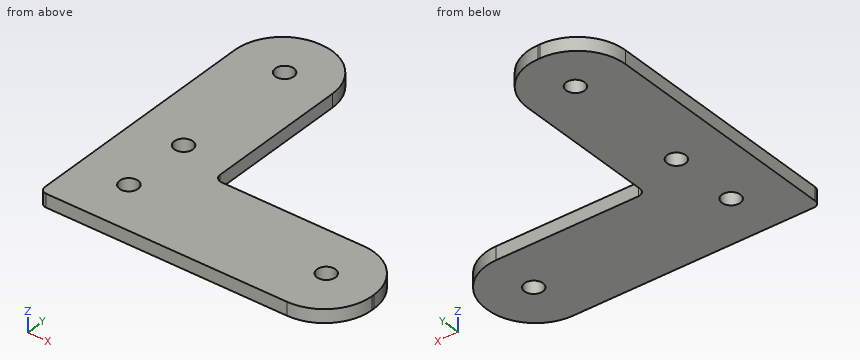
from build123d import *

# Parameters (mm, degrees)
BOSS_EXTRUDE1_DEPTH      = 3
FILLET4_R                = 21.5
FILLET5_R                = 3.4
FILLET6_R                = 3
F_5_16_CLEARANCE_HOLE1_D = 8.3185


with BuildPart() as part:
    # Sketch1 → Boss-Extrude1 (new, symmetric)
    with BuildSketch(Plane.XY):
        Polygon((0, 133), (0, 0), (133, 0), (133, 44), (44, 44), (44, 133), align=None)
    extrude(amount=BOSS_EXTRUDE1_DEPTH, both=True)

    # Fillet4
    fillet4_edges = [part.edges().sort_by_distance(p)[0] for p in [
        (133, 44, 0),
        (133, 0, 0),
        (0, 133, 0),
        (44, 133, 0),
    ]]
    fillet(fillet4_edges, radius=FILLET4_R)

    # Fillet5
    fillet5_edges = [part.edges().sort_by_distance(p)[0] for p in [
        (44, 44, 0),
    ]]
    fillet(fillet5_edges, radius=FILLET5_R)

    # Fillet6
    fillet6_edges = [part.edges().sort_by_distance(p)[0] for p in [
        (0, 0, 0),
    ]]
    fillet(fillet6_edges, radius=FILLET6_R)

    # 5/16 Clearance Hole1 (through all)
    with Locations(Plane.XY.offset(3)):
        with Locations((22.5, 111.5), (22.5, 53.7884), (22.5, 22.5), (111.5, 22.5)):
            Hole(F_5_16_CLEARANCE_HOLE1_D / 2)


solid = part.part
Model file for the job. Use its own axes, mm. Coordinates: 2 decimals unless noted, no trailing zeros. Write each loop counter-clockwise with the first axis right and the second up, starting at its lowest first coordinate (ties: lowest second). Pieces come first, ordered by that corner, then holes. Notation, with made-up numbers: (-8, -11.75) - (43, -11.75) arc R30 ccw to (43, 15.25) - close; hole circle Ø10 at (-5.75, 26.5). An arc over 180 degrees is marked (long way). Write each question's results on one line, items separated by ' | '. Start each with the question number.
1) Cut at B-B (y = 80). Write the cut outline in (x, z).
2) Flat gauge pins, fed straight in: P1, Ø9.5, axis at x = 22.5, y = 22.5, coming from the -Z side; P2, Ø2, axis at x = 26, z = 0.5, coming from the +Y side; P3, Ø3, axis at x = 70, z = -2, coming from the +Y side; P4, Ø6.5, axis at x = 22.5, y = 53.79, coming from the -Z side. Where does each tip first touch, or does it go through?
3) Cut at C-C (x = 34). Write the cut outline in (y, z), then the cut area to 3 significant figures.
4) Cut at A-A (z = 0.3). Write the cut outline in (x, y), then the cut area to 3 significant figures.
5) Probe line 1 along X through (y, z) = (63, -2.5); line 2 along X through (y, z) = (34.5, 1.7). List the from-to ranges inside material, lowest first. Write a range as from..to.
Returned:
1) outline: (0, -3) - (44, -3) - (44, 3) - (0, 3) - close
2) P1: z = -3 | P2: y = 132.85 | P3: y = 44 | P4: through
3) outline: (0, -3) - (129.67, -3) - (129.67, 3) - (0, 3) - close | area: 778 mm^2
4) outline: (0, 3) arc R3 ccw to (3, 0) - (111.5, 0) arc R21.5 ccw to (133, 21.5) - (133, 22.5) arc R21.5 ccw to (111.5, 44) - (47.4, 44) arc R3.4 cw to (44, 47.4) - (44, 111.5) arc R21.5 ccw to (22.5, 133) - (21.5, 133) arc R21.5 ccw to (0, 111.5) - close; hole circle Ø8.32 at (22.5, 22.5); hole circle Ø8.32 at (22.5, 53.79); hole circle Ø8.32 at (22.5, 111.5); hole circle Ø8.32 at (111.5, 22.5) | area: 9,150 mm^2
5) line 1: 0..44 | line 2: 0..129.34
